Build history of the part. All positions in model axes, mm. A direction names the side the tool comes from. Round coordinates to 2 decimals unless told otherwise and drop trailing zeros. Loops run counter-clockwise (first coordinate to the right, second up) from the corner with the lowest first, then second, coordinate; pieces in that order, holes last. Notation, with made-up numbers: (-25, 89) - (0, 89) arc R20 ccw to (0, 116) - close; hole circle Ø7 at (-34, -29). An arc over 180 degrees is marked (long way). Use a Markdown table: item, result.
from build123d import *

# Parameters (mm, degrees)
PCB_EDGE_SUPPORT_DEPTH       = 3
SKETCH_2_R                   = 3.5
PCB_SCREW_LANDS_DEPTH        = 3
SKETCH_3_W                   = 6.975
SKETCH_3_H                   = 4
SKETCH_3_W_2                 = 5.975
FLOATING_MOUNT_BRIDGES_DEPTH = 3
SKETCH_4_R                   = 4
SKETCH_4_R_2                 = 3.4
FLOATING_MOUNT_EARS_DEPTH    = 3
SKETCH_5_R                   = 1.15
PCB_M2_CLEARANCE_DEPTH       = 4
SKETCH_6_R                   = 1.7
M2_ADJUSTMENT_0P7_DEPTH      = 4


with BuildPart() as part:
    # 草图1 → PCB_edge_support (new body)
    with BuildSketch(Plane.XY):
        with BuildLine():
            Line((1, -0.5), (23.05, -0.5))
            ThreePointArc((23.05, -0.5), (24.110660172, -0.060660172), (24.55, 1))
            Line((24.55, 1), (24.55, 34.73))
            ThreePointArc((24.55, 34.73), (24.110660172, 35.790660172), (23.05, 36.23))
            Line((23.05, 36.23), (1, 36.23))
            ThreePointArc((1, 36.23), (-0.060660172, 35.790660172), (-0.5, 34.73))
            Line((-0.5, 34.73), (-0.5, 1))
            ThreePointArc((-0.5, 1), (-0.060660172, -0.060660172), (1, -0.5))
        make_face()
        with BuildLine():
            Line((2.5, 1.5), (21.55, 1.5))
            ThreePointArc((21.55, 1.5), (22.257106781, 1.792893219), (22.55, 2.5))
            Line((22.55, 2.5), (22.55, 33.23))
            ThreePointArc((22.55, 33.23), (22.257106781, 33.937106781), (21.55, 34.23))
            Line((21.55, 34.23), (2.5, 34.23))
            ThreePointArc((2.5, 34.23), (1.792893219, 33.937106781), (1.5, 33.23))
            Line((1.5, 33.23), (1.5, 2.5))
            ThreePointArc((1.5, 2.5), (1.792893219, 1.792893219), (2.5, 1.5))
        make_face(mode=Mode.SUBTRACT)
    extrude(amount=PCB_EDGE_SUPPORT_DEPTH)

    # 草图2 → PCB_screw_lands (add)
    with BuildSketch(Plane.XY):
        with Locations((3.5, 3.36)):
            Circle(SKETCH_2_R)
        with Locations((20.55, 3.36)):
            Circle(SKETCH_2_R)
    extrude(amount=PCB_SCREW_LANDS_DEPTH)

    # 草图3 → Floating_mount_bridges (add)
    with BuildSketch(Plane.XY):
        with Locations((-1.4875, 8.62)):
            Rectangle(SKETCH_3_W, SKETCH_3_H)
        with Locations((25.0375, 28.62)):
            Rectangle(SKETCH_3_W_2, SKETCH_3_H)
    extrude(amount=FLOATING_MOUNT_BRIDGES_DEPTH)

    # 草图4 → Floating_mount_ears (add)
    with BuildSketch(Plane.XY):
        with Locations((-4.975, 8.62)):
            Circle(SKETCH_4_R)
        with Locations((28.325, 28.62)):
            Circle(SKETCH_4_R_2)
    extrude(amount=FLOATING_MOUNT_EARS_DEPTH)

    # 草图5 → PCB_M2_clearance (cut)
    with BuildSketch(Plane.XY):
        with Locations((3.5, 3.36)):
            Circle(SKETCH_5_R)
        with Locations((20.55, 3.36)):
            Circle(SKETCH_5_R)
    extrude(amount=PCB_M2_CLEARANCE_DEPTH, mode=Mode.SUBTRACT)

    # 草图6 → M2_adjustment_0p7 (cut)
    with BuildSketch(Plane.XY):
        with Locations((-4.975, 8.62)):
            Circle(SKETCH_6_R)
        with Locations((28.325, 28.62)):
            Circle(SKETCH_6_R)
    extrude(amount=M2_ADJUSTMENT_0P7_DEPTH, mode=Mode.SUBTRACT)


solid = part.part
Q1. Probe line 1 (X direction, y = 3.36, z = 1.7); line 2 (Y direction, x = 3.5, z = 2.05); line 3 (Y direction, x = 4.5, z = 2.65). List the from-to ranges inside material, lowest first.
Results found:
| item | result |
|---|---|
| line 1 | x = -0.5 to 2.35, 4.65 to 7, 17.05 to 19.4, 21.7 to 24.55 |
| line 2 | y = -0.5 to 2.21, 4.51 to 6.86, 34.23 to 36.23 |
| line 3 | y = -0.5 to 2.79, 3.93 to 6.71, 34.23 to 36.23 |
Q2. Pull direction X, two halves, no side cores. Call faces 1 (the face through (24.1, -0.07, 1.48)), 2 (the face through (3.251, 2.237, 1.479)), 3 (the face through (-0.05, 35.8, 1.48)): pulls with the +X half, pulls with the -X half, needs draft (parallel to the pull), parting line crosses it, or undercut.
Results found:
| item | result |
|---|---|
| face 1 | pulls with the +X half |
| face 2 | undercut |
| face 3 | pulls with the -X half |
Q3. Cut at D-D, the plane x = 14. List the corners of the cut face in (y, z).
Results found:
| item | result |
|---|---|
| outline | (-0.5, 0) - (1.5, 0) - (1.5, 3) - (-0.5, 3) - close; (34.23, 0) - (36.23, 0) - (36.23, 3) - (34.23, 3) - close |
Q4. Cut at A-A, the plane x = 20.55. List the corners of the cut face in (y, z).
Results found:
| item | result |
|---|---|
| outline | (-0.5, 0) - (2.21, 0) - (2.21, 3) - (-0.5, 3) - close; (4.51, 0) - (6.86, 0) - (6.86, 3) - (4.51, 3) - close; (34.23, 0) - (36.23, 0) - (36.23, 3) - (34.23, 3) - close |
Q5. Cut at B-B, the plane y = 16.5. List the corners of the cut face in (x, z), plus the area to 3 significant figures.
Results found:
| item | result |
|---|---|
| outline | (-0.5, 0) - (1.5, 0) - (1.5, 3) - (-0.5, 3) - close; (22.55, 0) - (24.55, 0) - (24.55, 3) - (22.55, 3) - close |
| area | 12.0 mm2 |
Q6. Which spindle directions (+Z, -Z, +X, -X, +Y, -Y) get a long thin tool onto all of the face, cutting with end or side? Do faces 4 (the face through (25, 30.62, 1)), 5 (the face through (12, 34.23, 1)), 6 (the face through (24.1, 35.8, 1.5)). Say none if no direction does.
Results found:
| item | result |
|---|---|
| face 4 | +Z, -Z, +Y |
| face 5 | +Z, -Z |
| face 6 | +Z, -Z, +X, +Y |
Q7. Cut at C-C, the plane y = 8.62. List the corners of the cut face in (x, z) (3 decimals).
Results found:
| item | result |
|---|---|
| outline | (-8.975, 0) - (-6.675, 0) - (-6.675, 3) - (-8.975, 3) - close; (-3.275, 0) - (2, 0) - (2, 3) - (-3.275, 3) - close; (22.55, 0) - (24.55, 0) - (24.55, 3) - (22.55, 3) - close |
Q8. Drop flat-ended pins along their axis: pin 1 (1 mm diameter, centred on y = 25.5, z = 2, fed in from +X); pin 2 (1.5 mm diameter, centred on y = 9.5, z = 0.5, fed in from -X); pin 3 (0.8 mm diameter, centred on x = -1, z = 1.5, fed in from -Y). Give the stop position or say it passes through.
Results found:
| item | result |
|---|---|
| pin 1 | stops at x = 30.49 |
| pin 2 | stops at x = -8.97 |
| pin 3 | stops at y = 6.62 |
